from build123d import *

# Parameters (mm, degrees)
PAD_DEPTH       = 25
SKETCH001_R     = 1.5
PAD001_DEPTH    = 6
SKETCH002_R     = 1.5
POCKET_DEPTH    = 8.5
CHAMFER_SIZE    = 1.5
CHAMFER001_SIZE = 0.5


with BuildPart() as part:
    # Sketch → Pad (new body)
    with BuildSketch(Plane.XY):
        Polygon((-2.75, -1.587713), (-2.75, 1.587713), (0, 3.175426), (2.75, 1.587713), (2.75, -1.587713), (0, -3.175426), align=None)
    extrude(amount=PAD_DEPTH)

    # Sketch001 (on Face7 of Pad) → Pad001 (new body)
    with BuildSketch(Plane(origin=(0, 0, 0), x_dir=(1, 0, 0), z_dir=(0, 0, -1))):
        Circle(SKETCH001_R)
    extrude(amount=PAD001_DEPTH)

    # Sketch002 (on Face5 of Pad001) → Pocket (cut)
    with BuildSketch(Plane.XY.offset(25)):
        Circle(SKETCH002_R)
    extrude(amount=-POCKET_DEPTH, mode=Mode.SUBTRACT)

    # Chamfer
    chamfer_edges = [part.edges().sort_by_distance(p)[0] for p in [
        (-1.5, 0, 16.5),
    ]]
    chamfer(chamfer_edges, length=CHAMFER_SIZE)

    # Chamfer001
    chamfer001_edges = [part.edges().sort_by_distance(p)[0] for p in [
        (-1.5, 0, -6),
    ]]
    chamfer(chamfer001_edges, length=CHAMFER001_SIZE)


solid = part.part
The listing builds one solid part. Answer for the finished solid, in the listing's coordinates (mm). A direction names the side the tool comes from. Coordinates: 2 decimals unless noted, no trailing zeros. Write each loop counter-clockwise with the first axis right and the second up, starting at its lowest first coordinate (ties: lowest second). Pieces come first, ordered by that corner, then holes. Notation, with made-up numbers: (21, 82) - (33, 82) arc R23 ccw to (33, 104) - close; hole circle Ø7 at (22, 53.5). An arc over 180 degrees is marked (long way). Put each result on its own line as item: value.
1. The part is cut by section A-A on z = 21.5. Give the vertices of the cut face in (x, y), plus the area to 3 significant figures.
Answer sheet:
outline: (-2.75, -1.59) - (0, -3.18) - (2.75, -1.59) - (2.75, 1.59) - (0, 3.18) - (-2.75, 1.59) - close; hole circle Ø3 at (0, 0)
area: 19.1 mm^2
2. A tool of negligible diameter and unlimited length cuts with its end or side. For faces 1 (the face through (-1.5, -0.07, -2.71)), 2 (the face through (-2.75, 0, 12)), from which of +Z, -Z, +X, -X, +Y, -Y can it reach the whole face along a straight path? Write none if from no direction.
Answer sheet:
face 1: -Z
face 2: +Z, -Z, -X, +Y, -Y
3. Determine the mould class of faces 3 (the face through (-0.322, -0.247, 16.906)), 4 (the face through (1.36, 2.39, 12.32)), 5 (the face through (-1.5, 0.07, 21.55)), 6 (the face through (1.3, -1.4, 0)) for opening direction Y: pulls with the +Y half, pulls with the -Y half, needs draft (parallel to the pull), parting line crosses it, or undercut.
Answer sheet:
face 3: undercut
face 4: pulls with the +Y half
face 5: undercut
face 6: needs draft
4. The part is cut by section C-C on y = 2.25. Give the vertices of the cut face in (x, z).
Answer sheet:
outline: (-1.6, 0) - (1.6, 0) - (1.6, 25) - (-1.6, 25) - close
5. Flat-ended cylindrical pins translate along their axes: pin 1 Ø1.5 at (x, y) = (-1, 2.5) entering from -Z; pin 2 Ø1 at (x, y) = (0.5, -1.5) entering from -Z; pin 3 Ø1.5 at (x, z) = (2, 15.5) entering from -Y. Find the tip coordinate at first contact, or state that the pin passes through.
Answer sheet:
pin 1: stops at z = 0
pin 2: stops at z = -5.92
pin 3: stops at y = -2.45
6. The part is cut by section B-B on z = 1. Give the vertices of the cut face in (x, y), plus the area to 3 significant figures.
Answer sheet:
outline: (-2.75, -1.59) - (0, -3.18) - (2.75, -1.59) - (2.75, 1.59) - (0, 3.18) - (-2.75, 1.59) - close
area: 26.2 mm^2
7. Find the intervals of material crossed by line 1 along Z through (x, y) = (-0.1, -2); line 2 along Y through (x, z) = (-1, 22); line 3 along X through (y, z) = (0.25, 23), in increasing order. Write a range as from..to.
Answer sheet:
line 1: z = 0..25
line 2: y = -2.6..-1.12, 1.12..2.6
line 3: x = -2.75..-1.48, 1.48..2.75
8. The part is cut by section D-D on x = -2.05. Give the vertices of the cut face in (y, z), plus the area to 3 significant figures.
Answer sheet:
outline: (-1.99, 0) - (1.99, 0) - (1.99, 25) - (-1.99, 25) - close
area: 99.6 mm^2
